from build123d import *

# Parameters (mm, degrees)
F1_DEPTH = 100
F2_W     = 37.5
F2_H     = 37.5
F2_R     = 10
F3_DEPTH = 45
F4_W     = 200
F4_H     = 15
F5_DEPTH = 15
F6_R     = 2.5
F7_DEPTH = 200
F8_R     = 15


# Not quite as in the source:
# - a feature of the source that left no trace in its solid (it failed there, or was rolled back) is left out


with BuildPart() as f1:
    # F0 (on Top) → F1 (new body)
    with BuildSketch(Plane.XY):
        Polygon((137.5, 225), (-137.5, 225), (-137.5, -225), (-100, -225), (-100, -105), (100, -105), (100, -225), (137.5, -225), align=None)
    extrude(amount=F1_DEPTH)

    # F2 (on face) → F3 (cut)
    with BuildSketch(Plane(origin=(0, 0, 0), x_dir=(1, 0, 0), z_dir=(0, 0, -1))):
        with Locations((-118.75, 206.25)):
            Rectangle(F2_W, F2_H)
        with Locations((-118.75, 206.25)):
            Circle(F2_R, mode=Mode.SUBTRACT)
    extrude(amount=-F3_DEPTH, mode=Mode.SUBTRACT)

    # F4 (on face) → F5 (cut)
    with BuildSketch(Plane.XZ.offset(105)):
        with Locations((0, 7.5)):
            Rectangle(F4_W, F4_H)
    extrude(amount=-F5_DEPTH, mode=Mode.SUBTRACT)

    # F6 (on face) → F7 (join)
    with BuildSketch(Plane.YZ.offset(-100)):
        with Locations((-97.5, 7.5)):
            Circle(F6_R)
    extrude(amount=F7_DEPTH)

    # F8
    f8_edges = [f1.edges().sort_by_distance(p)[0] for p in [
        (118.75, -225, 0),
        (137.5, 0, 0),
        (-137.5, 18.75, 0),
        (-118.75, -187.5, 0),
    ]]
    fillet(f8_edges, radius=F8_R)


solid = f1.part
The model under review builds one solid part; all positions refer to its coordinate system, in mm. A direction names the side the tool comes from. Give positions to 0.01 mm unless a question says otherwise; leave off trailing zeros. Write each loop counter-clockwise with the first axis right and the second up, starting at its lowest first coordinate (ties: lowest second). Pieces come first, ordered by that corner, then holes.
1. Draft analysis for pull direction Y (two halves, no side actions). For faces 1 (the flat face through (2, 225, 49)), 2 (the flat face through (-127, -215, 45)), 3 (the flat face through (-119, -206, 0)), 4 (the flat face through (-1, -105, 57)), state which applies: +Y half, -Y half, draft (parallel to the pull), parting line (faces both ways), or undercut.
2. For P1, Ø7.5, axis at x = -4, z = 8.5, coming from the -Y side; P2, Ø3, axis at x = -53.5, z = 15, coming from the -Y side; P3, Ø15, axis at x = -124.5, z = 35.5, coming from the -Y side, all flat-tipped, find the tip position at first contact; note any pin that passes through.
3. Add section C-C, the plane z = 64. Write out the cut boundary in (x, y).
4. Add section A-A, the plane y = -140. Write out the cut boundary in (x, z).
5. Tool access review of faces 5 (the cylindrical face through (-114.32, -182.99, 4.28)), 6 (the cylindrical face through (-128.74, -206.69, 22.18)), 7 (the cylindrical face through (-133.22, 15.86, 4.51)), 8 (the flat face through (-1, -98, 15)): name each direction out of +Z, -Z, +X, -X, +Y, -Y from which nothing blocks a thin tool from reaching the whole face with its end or side.
6. Add section B-B, the plane x = -84. Write out the cut boundary in (y, z), plus the area to 3 significant figures.
7. Wall thickness on L1, parallel to X at y = -154, z = 28.5; L2, parallel to Y at x = 0, z = 77; L3, parallel to Y at x = -122, z = 26: over which ranges is each line inside the solid? List them lowest first.
Worked answers:
1. face 1: +Y half
1. face 2: undercut
1. face 3: draft
1. face 4: -Y half
2. P1: stops at y = -100
2. P2: stops at y = -105
2. P3: stops at y = -216.25
3. outline: (-137.5, -225) - (-100, -225) - (-100, -105) - (100, -105) - (100, -225) - (137.5, -225) - (137.5, 225) - (-137.5, 225) - close
4. outline: (-137.5, 15) arc R15 ccw to (-122.5, 0) - (-100, 0) - (-100, 100) - (-137.5, 100) - close; (100, 0) - (122.5, 0) arc R15 ccw to (137.5, 15) - (137.5, 100) - (100, 100) - close
5. face 5: -Z, -X
5. face 6: -Z
5. face 7: -Z, -X, +Y
5. face 8: -Y
6. outline: (-105, 15) - (-90, 15) - (-90, 0) - (225, 0) - (225, 100) - (-105, 100) - close; circle Ø5 at (-97.5, 7.5)
6. area: 32,800 mm2
7. L1: x = -137.5 to -100, 100 to 137.5
7. L2: y = -105 to 225
7. L3: y = -215.71 to -196.79, -187.5 to 225
